from build123d import *

# Parameters (mm, degrees)
SKETCH1_R           = 3
BOSS_EXTRUDE1_DEPTH = 1.2
SKETCH2_R           = 0.9
SKETCH2_W           = 1.8
SKETCH2_H           = 1.2
CUT_EXTRUDE1_DEPTH  = 2.2
SKETCH3_R           = 0.701713619
SKETCH3_W           = 1
SKETCH3_H           = 1.403427238
CUT_EXTRUDE2_DEPTH  = 10


with BuildPart() as part:
    # Sketch1 → Boss-Extrude1 (new body)
    with BuildSketch(Plane.XY):
        with BuildLine():
            Line((-7.575, -3.856082857), (-7.575, -11.5))
            Line((-7.575, -11.5), (7.575, -11.5))
            Line((7.575, -11.5), (7.575, -3.856082857))
            ThreePointArc((7.575, -3.856082857), (7.994413326, -2.887794239), (8.290619699, -1.875))
            Line((8.290619699, -1.875), (8.5, -1.875))
            Line((8.5, -1.875), (8.5, 1.875))
            Line((8.5, 1.875), (8.290619699, 1.875))
            ThreePointArc((8.290619699, 1.875), (0, 8.5), (-8.290619699, 1.875))
            Line((-8.290619699, 1.875), (-8.5, 1.875))
            Line((-8.5, 1.875), (-8.5, -1.875))
            Line((-8.5, -1.875), (-8.290619699, -1.875))
            ThreePointArc((-8.290619699, -1.875), (-7.994413326, -2.887794239), (-7.575, -3.856082857))
        make_face()
        Circle(SKETCH1_R, mode=Mode.SUBTRACT)
    extrude(amount=BOSS_EXTRUDE1_DEPTH)

    # Sketch2 → Cut-Extrude1 (cut, through all)
    with BuildSketch(Plane.XY.offset(1.2)):
        with Locations((0, -8.5)):
            Circle(SKETCH2_R)
        with Locations((5.12, -8.5)):
            Circle(SKETCH2_R)
        with Locations((-5.12, -8.5)):
            Circle(SKETCH2_R)
        with Locations((5.12, -10.9)):
            Rectangle(SKETCH2_W, SKETCH2_H)
        with Locations((0, -10.9)):
            Rectangle(SKETCH2_W, SKETCH2_H)
        with Locations((-5.12, -10.9)):
            Rectangle(SKETCH2_W, SKETCH2_H)
        Polygon((7.575, -11.5), (7.575, -10.5), (6.575, -11.5), align=None)
        Polygon((-6.575, -11.5), (-7.575, -11.5), (-7.575, -10.5), align=None)
    extrude(amount=-CUT_EXTRUDE1_DEPTH, mode=Mode.SUBTRACT)

    # Sketch3 → Cut-Extrude2 (cut)
    with BuildSketch(Plane.XY.offset(1.2)):
        with Locations((8, 0)):
            Circle(SKETCH3_R)
        with Locations((-8, 0)):
            Circle(SKETCH3_R)
        with BuildLine():
            Line((7.287029985, 2.15851662), (9.119724122, 2.701385355))
            Line((9.119724122, 2.701385355), (8.018790887, 4.818175656))
            Line((8.018790887, 4.818175656), (6.514471485, 3.914289369))
            ThreePointArc((6.514471485, 3.914289369), (6.956367241, 3.060874843), (7.287029985, 2.15851662))
        make_face()
        with BuildLine():
            Line((8.018790887, -4.818175656), (9.119724122, -2.701385355))
            Line((9.119724122, -2.701385355), (7.287029985, -2.15851662))
            ThreePointArc((7.287029985, -2.15851662), (6.956367241, -3.060874843), (6.514471485, -3.914289369))
            Line((6.514471485, -3.914289369), (8.018790887, -4.818175656))
        make_face()
        with BuildLine():
            Line((-7.287029985, -2.15851662), (-9.119724122, -2.701385355))
            Line((-9.119724122, -2.701385355), (-8.018790887, -4.818175656))
            Line((-8.018790887, -4.818175656), (-6.514471485, -3.914289369))
            ThreePointArc((-6.514471485, -3.914289369), (-6.956367241, -3.060874843), (-7.287029985, -2.15851662))
        make_face()
        with BuildLine():
            Line((-8.018790887, 4.818175656), (-9.119724122, 2.701385355))
            Line((-9.119724122, 2.701385355), (-7.287029985, 2.15851662))
            ThreePointArc((-7.287029985, 2.15851662), (-6.956367241, 3.060874843), (-6.514471485, 3.914289369))
            Line((-6.514471485, 3.914289369), (-8.018790887, 4.818175656))
        make_face()
        with Locations((-8.5, 0)):
            Rectangle(SKETCH3_W, SKETCH3_H)
        with Locations((8.5, 0)):
            Rectangle(SKETCH3_W, SKETCH3_H)
    extrude(amount=-CUT_EXTRUDE2_DEPTH, mode=Mode.SUBTRACT)


solid = part.part
The listing builds one solid part. Answer for the finished solid, in the listing's coordinates (mm). A direction names the side the tool comes from. Coordinates: 2 decimals unless noted, no trailing zeros. Loops run counter-clockwise (first coordinate to the right, second up) from the corner with the lowest first, then second, coordinate; pieces in that order, holes last. Notation, with made-up numbers: (77, 64) -> (127, 64) arc R13 ccw to (127, 82) -> close; hole circle Ø1 at (50, -40). An arc over 180 degrees is marked (long way). Answer in a Markdown table with one row per item. Add a question column.
1. The part is cut by section D-D, the plane y = 1.5. Write down the section's boundary in (x, z), then the cut area to 3 significant figures.
2. Consider line 1 (Y direction, x = 0, z = 0.6); line 2 (X direction, y = -6, z = 0.5) (3 decimals); line 3 (Y direction, x = 7.75, z = 0.65). Determine where each line is inside the solid, lowest interval first. Write a range as [from, to].
3. The part is cut by section B-B, the plane x = 0. Write down the section's boundary in (y, z).
4. The part is cut by section A-A, the plane y = -8.5. Write down the section's boundary in (x, z) (3 decimals).
5. For faces 1 (the flat face through (-7.725, 2.288, 0.608)), 2 (the flat face through (-5, -10.3, 1)), 3 (the flat face through (-7.052, -4.237, 0.608)), 4 (the flat face through (-7.712, -2.285, 0.608)), 5 (the flat face through (0, -4, 1.2)), determine the directions among +Z, -Z, +X, -X, +Y, -Y from which every point of the face is accessible in a straight line to the end or side of a thin tool.
6. The part is cut by section C-C, the plane x = 5.12. Write down the section's boundary in (y, z), then the cut area to 3 significant figures.
Answer below:
| question | item | result |
|---|---|---|
| 1 | outline | (-8.5, 0) -> (-2.6, 0) -> (-2.6, 1.2) -> (-8.5, 1.2) -> close; (2.6, 0) -> (8.5, 0) -> (8.5, 1.2) -> (2.6, 1.2) -> close |
| 1 | area | 14.2 mm2 |
| 2 | line 1 | [-10.3, -9.4], [-7.6, -3], [3, 8.5] |
| 2 | line 2 | [-7.575, 7.575] |
| 2 | line 3 | [-2.3, -0.66], [0.66, 2.3] |
| 3 | outline | (-10.3, 0) -> (-9.4, 0) -> (-9.4, 1.2) -> (-10.3, 1.2) -> close; (-7.6, 0) -> (-3, 0) -> (-3, 1.2) -> (-7.6, 1.2) -> close; (3, 0) -> (8.5, 0) -> (8.5, 1.2) -> (3, 1.2) -> close |
| 4 | outline | (-7.575, 0) -> (-6.02, 0) -> (-6.02, 1.2) -> (-7.575, 1.2) -> close; (-4.22, 0) -> (-0.9, 0) -> (-0.9, 1.2) -> (-4.22, 1.2) -> close; (0.9, 0) -> (4.22, 0) -> (4.22, 1.2) -> (0.9, 1.2) -> close; (6.02, 0) -> (7.575, 0) -> (7.575, 1.2) -> (6.02, 1.2) -> close |
| 5 | face 1 | +Z, -Z, +Y |
| 5 | face 2 | +Z, -Z, -Y |
| 5 | face 3 | +Z, -Z, -X |
| 5 | face 4 | +Z, -Z |
| 5 | face 5 | +Z, +X, -X, +Y, -Y |
| 6 | outline | (-10.3, 0) -> (-9.4, 0) -> (-9.4, 1.2) -> (-10.3, 1.2) -> close; (-7.6, 0) -> (6.78, 0) -> (6.78, 1.2) -> (-7.6, 1.2) -> close |
| 6 | area | 18.3 mm2 |
